Here's how the part is built. I have some questions about the finished solid (model axes, mm). A direction names the side the tool comes from. Round coordinates to 2 decimals unless told otherwise and drop trailing zeros. Order: outer loops, then holes, each group sorted by start corner. A loop starts at its lowest first (then second) coordinate and runs counter-clockwise, first axis right, second up. Notation, with made-up numbers: M 44,35.5 L 78,35.5 A23 ccw 78,74.5 Z; hole C -11.75,37 d9. An arc over 180 degrees is marked long. Write each question's results on one line, items separated by ' | '. Start each with the question number.
```python
from build123d import *

# Parameters (mm, degrees)
SKETCH1_W           = 86.5
SKETCH1_H           = 23
SKETCH1_R           = 1.1
BOSS_EXTRUDE1_DEPTH = 4.5
CUT_EXTRUDE1_DEPTH  = 2
SKETCH3_R           = 2.55
BOSS_EXTRUDE2_DEPTH = 4.5
SKETCH6_R           = 9
CUT_EXTRUDE3_DEPTH  = 1.95
FILLET1_R           = 3
FILLET2_R           = 1
FILLET3_R           = 1
BOSS_EXTRUDE3_DEPTH = 2
FILLET4_R           = 3


with BuildPart() as part:
    # Sketch1 → Boss-Extrude1 (new body)
    with BuildSketch(Plane.XY):
        Rectangle(SKETCH1_W, SKETCH1_H)
        with Locations((38.25, 6.5)):
            Circle(SKETCH1_R, mode=Mode.SUBTRACT)
        with Locations((38.25, -6.5)):
            Circle(SKETCH1_R, mode=Mode.SUBTRACT)
        with Locations((-38.25, -6.5)):
            Circle(SKETCH1_R, mode=Mode.SUBTRACT)
        with Locations((-38.25, 6.5)):
            Circle(SKETCH1_R, mode=Mode.SUBTRACT)
    extrude(amount=BOSS_EXTRUDE1_DEPTH)

    # Sketch2 → Cut-Extrude1 (cut)
    with BuildSketch(Plane(origin=(0, 0, 0), x_dir=(-1, 0, 0), z_dir=(0, 0, -1))):
        with BuildLine():
            Line((-5, 9.5), (-35.604248689, 9.5))
            ThreePointArc((-35.604248689, 9.5), (-34.508342613, 5.085786438), (-38.25, 2.5))
            Line((-38.25, 2.5), (-38.25, -2.5))
            ThreePointArc((-38.25, -2.5), (-34.508342613, -5.085786438), (-35.604248689, -9.5))
            Line((-35.604248689, -9.5), (-5, -9.5))
            Line((-5, -9.5), (-5, 9.5))
        make_face()
        with BuildLine():
            Line((35.604248689, 9.5), (5, 9.5))
            Line((5, 9.5), (5, -9.5))
            Line((5, -9.5), (35.604248689, -9.5))
            ThreePointArc((35.604248689, -9.5), (34.508342613, -5.085786438), (38.25, -2.5))
            Line((38.25, -2.5), (38.25, 2.5))
            ThreePointArc((38.25, 2.5), (34.508342613, 5.085786438), (35.604248689, 9.5))
        make_face()
    extrude(amount=-CUT_EXTRUDE1_DEPTH, mode=Mode.SUBTRACT)

    # Sketch3 → Boss-Extrude2 (add, symmetric)
    with BuildSketch(Plane(origin=(0, 0, 0), x_dir=(0, 0, -1), z_dir=(1, 0, 0))):
        with BuildLine():
            Line((-29.5, 8), (-4.5, 8))
            Line((-4.5, 8), (-4.5, -8))
            Line((-4.5, -8), (-29.5, -8))
            ThreePointArc((-29.5, -8), (-37.5, 0), (-29.5, 8))
        make_face()
        with Locations((-29.5, 0)):
            Circle(SKETCH3_R, mode=Mode.SUBTRACT)
    extrude(amount=BOSS_EXTRUDE2_DEPTH, both=True)

    # Sketch6 → Cut-Extrude3 (cut, symmetric)
    with BuildSketch(Plane(origin=(0, 0, 0), x_dir=(0, 0, -1), z_dir=(1, 0, 0))):
        with Locations((-29.5, 0)):
            Circle(SKETCH6_R)
    extrude(amount=CUT_EXTRUDE3_DEPTH, both=True, mode=Mode.SUBTRACT)

    # Fillet1
    fillet1_edges = [part.edges().sort_by_distance(p)[0] for p in [
        (4.5, 0, 4.5),
        (-4.5, 0, 4.5),
        (0, -8, 4.5),
        (0, 8, 4.5),
        (43.25, -11.5, 2.25),
        (-43.25, -11.5, 2.25),
        (-43.25, 11.5, 2.25),
        (43.25, 11.5, 2.25),
    ]]
    fillet(fillet1_edges, radius=FILLET1_R)

    # Fillet2
    fillet2_edges = [part.edges().sort_by_distance(p)[0] for p in [
        (1.95, 0, 20.5),
        (-1.95, 0, 20.5),
    ]]
    fillet(fillet2_edges, radius=FILLET2_R)

    # Fillet3
    fillet3_edges = [part.edges().sort_by_distance(p)[0] for p in [
        (35.604248689, -9.5, 1),
        (38.25, -2.5, 1),
        (38.25, 2.5, 1),
        (35.604248689, 9.5, 1),
        (5, 9.5, 1),
        (5, -9.5, 1),
        (-35.604248689, -9.5, 1),
        (-5, -9.5, 1),
        (-5, 9.5, 1),
        (-35.604248689, 9.5, 1),
        (-38.25, 2.5, 1),
        (-38.25, -2.5, 1),
    ]]
    fillet(fillet3_edges, radius=FILLET3_R)

    # Sketch7 → Boss-Extrude3 (add)
    with BuildSketch(Plane(origin=(4.5, 0, 0), x_dir=(0, 0, -1), z_dir=(1, 0, 0))):
        Polygon((-14.457460059, 1.316051715), (-17, 0), (-14.457460059, 0), align=None)
        Polygon((-14.457460059, 0), (-17, 0), (-14.457460059, -1.316051715), align=None)
        with BuildLine():
            Line((-14.457460059, 0), (-14.457460059, -1.316051715))
            ThreePointArc((-14.457460059, -1.316051715), (-14.414371854, -0.658652749), (-14.4, 0))
            Line((-14.4, 0), (-14.457460059, 0))
        make_face()
        with BuildLine():
            ThreePointArc((-14.4, 0), (-14.414371854, 0.658652749), (-14.457460059, 1.316051715))
            Line((-14.457460059, 1.316051715), (-14.457460059, 0))
            Line((-14.457460059, 0), (-14.4, 0))
        make_face()
    boss_extrude3 = extrude(amount=BOSS_EXTRUDE3_DEPTH)

    # Mirror1: Boss-Extrude3 across plane
    add(boss_extrude3.mirror(Plane(origin=(0, 0, 0), x_dir=(0, 0, 1), z_dir=(1, 0, 0))))

    # Fillet4
    # the kernel refuses this fillet: 3 mm, written as the material it adds along each edge
    with BuildSketch(Plane(origin=(4.5, 0, 29.5), x_dir=(0, -0.5274118729194984, -0.8496097435314327), z_dir=(0, -0.8496097435314327, 0.5274118729194984))) as fillet4_piece_1_section:
        with BuildLine():
            CenterArc((17.928427125, 3), FILLET4_R, 199.471220634, 70.528779366)
            Line((15.1, 2), (15.043431458, 1.98))
            ThreePointArc((15.043431458, 1.98), (15.04, 1), (15.04, 0))
            Line((15.04, 0), (15.1, -0.06))
            Line((15.1, -0.06), (17.928427125, -0.06))
            Line((17.928427125, -0.06), (17.928427125, 0))
        make_face()
    fillet4_piece_1 = revolve(axis=Axis((4.5, 0, 29.5), (1, 0, 0)), revolution_arc=63.661503438, mode=Mode.PRIVATE)
    fillet4_piece_1 = split(fillet4_piece_1, bisect_by=Plane(origin=(4.961847774, -1.372551705, 14.348305169), z_dir=(0, 0.888082932047281, -0.4596832668330496)), keep=Keep.TOP, mode=Mode.PRIVATE)
    fillet4_piece_1 = split(fillet4_piece_1, bisect_by=Plane(origin=(4.961847774, 1.372551598, 14.348305377), z_dir=(0, -0.8880829320471848, -0.4596832668332354)), keep=Keep.TOP, mode=Mode.PRIVATE)
    add(fillet4_piece_1)
    with BuildSketch(Plane(origin=(-4.5, 0, 29.5), x_dir=(0, -0.5274118729194984, -0.8496097435314327), z_dir=(0, -0.8496097435314327, 0.5274118729194984))) as fillet4_piece_2_section:
        with BuildLine():
            CenterArc((17.928427125, -3), FILLET4_R, 90, 70.528779366)
            Line((15.1, -2), (15.043431458, -1.98))
            ThreePointArc((15.043431458, -1.98), (15.04, -1), (15.04, 0))
            Line((15.04, 0), (15.1, 0.06))
            Line((15.1, 0.06), (17.928427125, 0.06))
            Line((17.928427125, 0.06), (17.928427125, 0))
        make_face()
    fillet4_piece_2 = revolve(axis=Axis((-4.5, 0, 29.5), (1, 0, 0)), revolution_arc=63.661503438, mode=Mode.PRIVATE)
    fillet4_piece_2 = split(fillet4_piece_2, bisect_by=Plane(origin=(-4.961847774, -1.372551705, 14.348305169), z_dir=(0, 0.888082932047281, -0.4596832668330496)), keep=Keep.TOP, mode=Mode.PRIVATE)
    fillet4_piece_2 = split(fillet4_piece_2, bisect_by=Plane(origin=(-4.961847774, 1.372551598, 14.348305377), z_dir=(0, -0.8880829320471848, -0.4596832668332354)), keep=Keep.TOP, mode=Mode.PRIVATE)
    add(fillet4_piece_2)


solid = part.part
```
(1) I want a section at B-B on y = 6.5. Give the number of separate pieces and of enclosed holes in the cut face, and give its area (3 significant figures).
(2) On a 3-axis mill with a long thin cutter (end or side, diameter ignored), from which of +Z, -Z, +X, -X, +Y, -Y can I reach the whole of each face in a straight line? I mean faces 1 (the flat face through (1.95, 0, 26)), 2 (the cylindrical face through (-42.39, 10.6, 2.28)), 3 (the flat face through (-20, 9.5, 1)). Say none if no direction works.
(3) Please list where these lines run through material, in increasing order: line 1 (Y direction, x = 38.25, z = 2.5); line 2 (X direction, y = 1, z = 34).
(4) If we mould it in two halves opening along Z, with no side actions, what happens to faces 4 (the cylindrical face through (42.39, 10.6, 2.28)), 5 (the cylindrical face through (5.4, -0.15, 5.36)), 6 (the cylindrical face through (3.243, -0.176, 37.498))? For each: pulls with the +Z half, pulls with the -Z half, needs draft (parallel to the pull), parting line crosses it, or undercut.
(5) I want a section at A-A on x = -14.5. Write out the boundary of the cut face in (y, z).
(6) I'm going to push flat-ended pins straight in: pin 1 Ø2.5 at (x, z) = (2, 18) entering from +Y; pin 2 Ø2 at (x, y) = (13, 1.5) entering from +Z; pin 3 Ø13 at (y, z) = (0, 29) entering from -X. Where does each tip first touch, or does it pass through?
(7) I want a section at C-C on z = 18.5. Write out the boundary of the cut face in (x, y).
(8) I want a section at D-D on x = -36. Write out the boundary of the cut face in (y, z).
Solutions:
1) separate pieces: 3 | enclosed holes: 0 | area: 481 mm^2
2) face 1: +Z | face 2: +Z, -Z, -X, +Y | face 3: -Z
3) line 1: -11.5 to -7.6, -5.4 to 5.4, 7.6 to 11.5 | line 2: -4.5 to -1.95, 1.95 to 4.5
4) face 4: needs draft | face 5: undercut | face 6: pulls with the +Z half
5) outline: M -11.5,0 L -9.5,0 L -9.5,2 L 9.5,2 L 9.5,0 L 11.5,0 L 11.5,4.5 L -11.5,4.5 Z
6) pin 1: y = 8 | pin 2: z = 4.5 | pin 3: x = -4.5
7) outline: M -4.5,-8 L 4.5,-8 L 4.5,8 L -4.5,8 Z
8) outline: M -11.5,0 L -3.19,0 L -3.19,2 L 3.19,2 L 3.19,0 L 11.5,0 L 11.5,4.5 L -11.5,4.5 Z
